Can you work these out from the model? Positions are in its coordinate system, mm. A direction names the side the tool comes from. Round coordinates to 2 decimals unless told otherwise and drop trailing zeros. Order: outer loops, then holes, each group sorted by start corner. A loop starts at its lowest first (then second) coordinate and runs counter-clockwise, first axis right, second up.
Q1. If we section it at B-B (x = 0): Please give me the cut outline in (y, z), plus the area to 3 significant figures.
Q2. If we section it at A-A (z = 0): Please give me the cut outline in (x, y), plus the area to 3 significant figures.
Q3. If I drill on line 1 (Z direction, x = 0, y = 53); line 2 (Z direction, x = 7.5, y = 71); line 3 (X direction, y = 12.5, z = -408), over which ranges is the centre line in solid material (lowest first)?
Q4. If we section it at C-C (y = 28): Count the separate pieces of the cut face and the enclosed holes in it, plus the area to 3 significant figures.
Q5. We'd pull the mould along Z, two halves only. Please class faces 1 (the face through (-309.9, 40.5, 247)), 2 (the face through (-365, 5, -97)), 3 (the face through (353.146, 0.243, 111.211)): pulls with the +Z half, pulls with the -Z half, needs draft (parallel to the pull), parting line crosses it, or undercut.
Q6. For faces 4 (the face through (101, 77, 365)), 5 (the face through (274.128, 76.05, 86.327)), which set-ups out of +Z, -Z, +X, -X, +Y, -Y let a thin tool reach every point of the face, with its end or its side?
Q7. Will these pins go through, and if not, where does the flat tip stop? P1, Ø2, axis at x = -261, y = 70.5, coming from the +Z side; P2, Ø1, axis at y = 21.5, z = 157, coming from the +X side; P3, Ø1.5, axis at y = 72.5, z = 202.5, coming from the -X side.
from build123d import *

# Parameters (mm, degrees)
CUT_EXTRUDE2_REACH = 147
SKETCH2_R          = 22


with BuildPart() as part:
    # Sketch1 → Revolve1 (revolve)
    with BuildSketch(Plane.XY):
        with BuildLine():
            Line((287.4, 150), (304.8, 150))
            Line((304.8, 150), (304.8, 130))
            Line((304.8, 130), (369.380900162, 79.543870957))
            ThreePointArc((369.380900162, 79.543870957), (372.862020012, 77.653777093), (376.768837866, 77))
            Line((376.768837866, 77), (445, 77))
            Line((445, 77), (445, 5))
            Line((445, 5), (375, 5))
            Line((375, 5), (370, 0))
            Line((370, 0), (287.4, 0))
            Line((287.4, 0), (287.4, 150))
        make_face()
    revolve(axis=Axis((0, 150, 0), (0, -1, 0)))

    # Sketch2 → Cut-Extrude2 (cut, up to next)
    with BuildSketch(Plane.XZ.offset(-5), mode=Mode.PRIVATE) as cut_extrude2_sk1:
        with Locations((0, 409)):
            Circle(SKETCH2_R)
    cut_extrude2_tool1 = extrude(cut_extrude2_sk1.sketch, amount=-CUT_EXTRUDE2_REACH, mode=Mode.PRIVATE) & part.part
    add(cut_extrude2_tool1.solids().sort_by_distance((0, 5, 409))[0], mode=Mode.SUBTRACT)
    # Sketch2 → Cut-Extrude2 (cut, up to next)
    with BuildSketch(Plane.XZ.offset(-5), mode=Mode.PRIVATE) as cut_extrude2_sk2:
        with Locations((126.387950699, 388.982115165)):
            Circle(SKETCH2_R)
    cut_extrude2_tool2 = extrude(cut_extrude2_sk2.sketch, amount=-CUT_EXTRUDE2_REACH, mode=Mode.PRIVATE) & part.part
    add(cut_extrude2_tool2.solids().sort_by_distance((126.387951, 5, 388.982115))[0], mode=Mode.SUBTRACT)
    # Sketch2 → Cut-Extrude2 (cut, up to next)
    with BuildSketch(Plane.XZ.offset(-5), mode=Mode.PRIVATE) as cut_extrude2_sk3:
        with Locations((240.404168188, 330.887950699)):
            Circle(SKETCH2_R)
    cut_extrude2_tool3 = extrude(cut_extrude2_sk3.sketch, amount=-CUT_EXTRUDE2_REACH, mode=Mode.PRIVATE) & part.part
    add(cut_extrude2_tool3.solids().sort_by_distance((240.404168, 5, 330.887951))[0], mode=Mode.SUBTRACT)
    # Sketch2 → Cut-Extrude2 (cut, up to next)
    with BuildSketch(Plane.XZ.offset(-5), mode=Mode.PRIVATE) as cut_extrude2_sk4:
        with Locations((330.887950699, 240.404168188)):
            Circle(SKETCH2_R)
    cut_extrude2_tool4 = extrude(cut_extrude2_sk4.sketch, amount=-CUT_EXTRUDE2_REACH, mode=Mode.PRIVATE) & part.part
    add(cut_extrude2_tool4.solids().sort_by_distance((330.887951, 5, 240.404168))[0], mode=Mode.SUBTRACT)
    # Sketch2 → Cut-Extrude2 (cut, up to next)
    with BuildSketch(Plane.XZ.offset(-5), mode=Mode.PRIVATE) as cut_extrude2_sk5:
        with Locations((388.982115165, 126.387950699)):
            Circle(SKETCH2_R)
    cut_extrude2_tool5 = extrude(cut_extrude2_sk5.sketch, amount=-CUT_EXTRUDE2_REACH, mode=Mode.PRIVATE) & part.part
    add(cut_extrude2_tool5.solids().sort_by_distance((388.982115, 5, 126.387951))[0], mode=Mode.SUBTRACT)
    # Sketch2 → Cut-Extrude2 (cut, up to next)
    with BuildSketch(Plane.XZ.offset(-5), mode=Mode.PRIVATE) as cut_extrude2_sk6:
        with Locations((409, 0)):
            Circle(SKETCH2_R)
    cut_extrude2_tool6 = extrude(cut_extrude2_sk6.sketch, amount=-CUT_EXTRUDE2_REACH, mode=Mode.PRIVATE) & part.part
    add(cut_extrude2_tool6.solids().sort_by_distance((409, 5, 0))[0], mode=Mode.SUBTRACT)
    # Sketch2 → Cut-Extrude2 (cut, up to next)
    with BuildSketch(Plane.XZ.offset(-5), mode=Mode.PRIVATE) as cut_extrude2_sk7:
        with Locations((388.982115165, -126.387950699)):
            Circle(SKETCH2_R)
    cut_extrude2_tool7 = extrude(cut_extrude2_sk7.sketch, amount=-CUT_EXTRUDE2_REACH, mode=Mode.PRIVATE) & part.part
    add(cut_extrude2_tool7.solids().sort_by_distance((388.982115, 5, -126.387951))[0], mode=Mode.SUBTRACT)
    # Sketch2 → Cut-Extrude2 (cut, up to next)
    with BuildSketch(Plane.XZ.offset(-5), mode=Mode.PRIVATE) as cut_extrude2_sk8:
        with Locations((330.887950699, -240.404168188)):
            Circle(SKETCH2_R)
    cut_extrude2_tool8 = extrude(cut_extrude2_sk8.sketch, amount=-CUT_EXTRUDE2_REACH, mode=Mode.PRIVATE) & part.part
    add(cut_extrude2_tool8.solids().sort_by_distance((330.887951, 5, -240.404168))[0], mode=Mode.SUBTRACT)
    # Sketch2 → Cut-Extrude2 (cut, up to next)
    with BuildSketch(Plane.XZ.offset(-5), mode=Mode.PRIVATE) as cut_extrude2_sk9:
        with Locations((240.404168188, -330.887950699)):
            Circle(SKETCH2_R)
    cut_extrude2_tool9 = extrude(cut_extrude2_sk9.sketch, amount=-CUT_EXTRUDE2_REACH, mode=Mode.PRIVATE) & part.part
    add(cut_extrude2_tool9.solids().sort_by_distance((240.404168, 5, -330.887951))[0], mode=Mode.SUBTRACT)
    # Sketch2 → Cut-Extrude2 (cut, up to next)
    with BuildSketch(Plane.XZ.offset(-5), mode=Mode.PRIVATE) as cut_extrude2_sk10:
        with Locations((126.387950699, -388.982115165)):
            Circle(SKETCH2_R)
    cut_extrude2_tool10 = extrude(cut_extrude2_sk10.sketch, amount=-CUT_EXTRUDE2_REACH, mode=Mode.PRIVATE) & part.part
    add(cut_extrude2_tool10.solids().sort_by_distance((126.387951, 5, -388.982115))[0], mode=Mode.SUBTRACT)
    # Sketch2 → Cut-Extrude2 (cut, up to next)
    with BuildSketch(Plane.XZ.offset(-5), mode=Mode.PRIVATE) as cut_extrude2_sk11:
        with Locations((0, -409)):
            Circle(SKETCH2_R)
    cut_extrude2_tool11 = extrude(cut_extrude2_sk11.sketch, amount=-CUT_EXTRUDE2_REACH, mode=Mode.PRIVATE) & part.part
    add(cut_extrude2_tool11.solids().sort_by_distance((0, 5, -409))[0], mode=Mode.SUBTRACT)
    # Sketch2 → Cut-Extrude2 (cut, up to next)
    with BuildSketch(Plane.XZ.offset(-5), mode=Mode.PRIVATE) as cut_extrude2_sk12:
        with Locations((-126.387950699, -388.982115165)):
            Circle(SKETCH2_R)
    cut_extrude2_tool12 = extrude(cut_extrude2_sk12.sketch, amount=-CUT_EXTRUDE2_REACH, mode=Mode.PRIVATE) & part.part
    add(cut_extrude2_tool12.solids().sort_by_distance((-126.387951, 5, -388.982115))[0], mode=Mode.SUBTRACT)
    # Sketch2 → Cut-Extrude2 (cut, up to next)
    with BuildSketch(Plane.XZ.offset(-5), mode=Mode.PRIVATE) as cut_extrude2_sk13:
        with Locations((-240.404168188, -330.887950699)):
            Circle(SKETCH2_R)
    cut_extrude2_tool13 = extrude(cut_extrude2_sk13.sketch, amount=-CUT_EXTRUDE2_REACH, mode=Mode.PRIVATE) & part.part
    add(cut_extrude2_tool13.solids().sort_by_distance((-240.404168, 5, -330.887951))[0], mode=Mode.SUBTRACT)
    # Sketch2 → Cut-Extrude2 (cut, up to next)
    with BuildSketch(Plane.XZ.offset(-5), mode=Mode.PRIVATE) as cut_extrude2_sk14:
        with Locations((-330.887950699, -240.404168188)):
            Circle(SKETCH2_R)
    cut_extrude2_tool14 = extrude(cut_extrude2_sk14.sketch, amount=-CUT_EXTRUDE2_REACH, mode=Mode.PRIVATE) & part.part
    add(cut_extrude2_tool14.solids().sort_by_distance((-330.887951, 5, -240.404168))[0], mode=Mode.SUBTRACT)
    # Sketch2 → Cut-Extrude2 (cut, up to next)
    with BuildSketch(Plane.XZ.offset(-5), mode=Mode.PRIVATE) as cut_extrude2_sk15:
        with Locations((-388.982115165, -126.387950699)):
            Circle(SKETCH2_R)
    cut_extrude2_tool15 = extrude(cut_extrude2_sk15.sketch, amount=-CUT_EXTRUDE2_REACH, mode=Mode.PRIVATE) & part.part
    add(cut_extrude2_tool15.solids().sort_by_distance((-388.982115, 5, -126.387951))[0], mode=Mode.SUBTRACT)
    # Sketch2 → Cut-Extrude2 (cut, up to next)
    with BuildSketch(Plane.XZ.offset(-5), mode=Mode.PRIVATE) as cut_extrude2_sk16:
        with Locations((-409, 0)):
            Circle(SKETCH2_R)
    cut_extrude2_tool16 = extrude(cut_extrude2_sk16.sketch, amount=-CUT_EXTRUDE2_REACH, mode=Mode.PRIVATE) & part.part
    add(cut_extrude2_tool16.solids().sort_by_distance((-409, 5, 0))[0], mode=Mode.SUBTRACT)
    # Sketch2 → Cut-Extrude2 (cut, up to next)
    with BuildSketch(Plane.XZ.offset(-5), mode=Mode.PRIVATE) as cut_extrude2_sk17:
        with Locations((-388.982115165, 126.387950699)):
            Circle(SKETCH2_R)
    cut_extrude2_tool17 = extrude(cut_extrude2_sk17.sketch, amount=-CUT_EXTRUDE2_REACH, mode=Mode.PRIVATE) & part.part
    add(cut_extrude2_tool17.solids().sort_by_distance((-388.982115, 5, 126.387951))[0], mode=Mode.SUBTRACT)
    # Sketch2 → Cut-Extrude2 (cut, up to next)
    with BuildSketch(Plane.XZ.offset(-5), mode=Mode.PRIVATE) as cut_extrude2_sk18:
        with Locations((-330.887950699, 240.404168188)):
            Circle(SKETCH2_R)
    cut_extrude2_tool18 = extrude(cut_extrude2_sk18.sketch, amount=-CUT_EXTRUDE2_REACH, mode=Mode.PRIVATE) & part.part
    add(cut_extrude2_tool18.solids().sort_by_distance((-330.887951, 5, 240.404168))[0], mode=Mode.SUBTRACT)
    # Sketch2 → Cut-Extrude2 (cut, up to next)
    with BuildSketch(Plane.XZ.offset(-5), mode=Mode.PRIVATE) as cut_extrude2_sk19:
        with Locations((-240.404168188, 330.887950699)):
            Circle(SKETCH2_R)
    cut_extrude2_tool19 = extrude(cut_extrude2_sk19.sketch, amount=-CUT_EXTRUDE2_REACH, mode=Mode.PRIVATE) & part.part
    add(cut_extrude2_tool19.solids().sort_by_distance((-240.404168, 5, 330.887951))[0], mode=Mode.SUBTRACT)
    # Sketch2 → Cut-Extrude2 (cut, up to next)
    with BuildSketch(Plane.XZ.offset(-5), mode=Mode.PRIVATE) as cut_extrude2_sk20:
        with Locations((-126.387950699, 388.982115165)):
            Circle(SKETCH2_R)
    cut_extrude2_tool20 = extrude(cut_extrude2_sk20.sketch, amount=-CUT_EXTRUDE2_REACH, mode=Mode.PRIVATE) & part.part
    add(cut_extrude2_tool20.solids().sort_by_distance((-126.387951, 5, 388.982115))[0], mode=Mode.SUBTRACT)


solid = part.part
Solution:
1. outline: (0, -370) - (5, -375) - (5, -387) - (77, -387) - (77, -376.77) arc R12 cw to (79.54, -369.38) - (130, -304.8) - (150, -304.8) - (150, -287.4) - (0, -287.4) - close; (0, 287.4) - (150, 287.4) - (150, 304.8) - (130, 304.8) - (79.54, 369.38) arc R12 cw to (77, 376.77) - (77, 387) - (5, 387) - (5, 375) - (0, 370) - close; (5, -445) - (77, -445) - (77, -431) - (5, -431) - close; (5, 431) - (77, 431) - (77, 445) - (5, 445) - close
1. area: 23,300 mm2
2. outline: (-445, 5) - (-431, 5) - (-431, 77) - (-445, 77) - close; (-387, 5) - (-375, 5) - (-370, 0) - (-287.4, 0) - (-287.4, 150) - (-304.8, 150) - (-304.8, 130) - (-369.38, 79.54) arc R12 cw to (-376.77, 77) - (-387, 77) - close; (287.4, 0) - (370, 0) - (375, 5) - (387, 5) - (387, 77) - (376.77, 77) arc R12 cw to (369.38, 79.54) - (304.8, 130) - (304.8, 150) - (287.4, 150) - close; (431, 5) - (445, 5) - (445, 77) - (431, 77) - close
2. area: 23,300 mm2
3. line 1: z = -445 to -431, -387 to -287.4, 287.4 to 387, 431 to 445
3. line 2: z = -444.94 to -429.68, -388.32 to -287.3, 287.3 to 388.32, 429.68 to 444.94
3. line 3: x = -177.65 to -137.45, -115.33 to -21.98, 21.98 to 115.33, 137.45 to 177.65
4. separate pieces: 1
4. enclosed holes: 21
4. area: 332,000 mm2
5. face 1: undercut
5. face 2: needs draft
5. face 3: parting line crosses it
6. face 4: +Y
6. face 5: +Y, -Y
7. P1: stops at z = 361.14
7. P2: stops at x = 416.57
7. P3: stops at x = -396.64
